Part model, mm, in its own coordinate system. A direction names the side the tool comes from. Coordinates: 2 decimals unless noted, no trailing zeros. Loops run counter-clockwise (first coordinate to the right, second up) from the corner with the lowest first, then second, coordinate; pieces in that order, holes last. Notation, with made-up numbers: (27, 35.25) - (62, 35.25) arc R22 cw to (62, 64.25) - close; hole circle Ø6 at (58.25, 54). An arc over 180 degrees is marked (long way). Use a Markdown table: item, result. Add a question column.
1. Wall check: probe 1 along X at (y, z) = (1.5, 0); probe 2 along Y at (x, z) = (5, 0.9); probe 3 along Y at (x, z) = (31.5, -2.6). Give the ranges that are in metal, low to high. Write a range as [from, to].
2. 3-axis set-ups, long thin cutter, end or side, ignore diameter. For faces 1 (the flat face through (16, 1, -3)), 2 (the flat face through (32, 3.5, 2)): which of +Z, -Z, +X, -X, +Y, -Y reach the whole face in a straight line?
3. Band-saw the part on C-C, the plane x = 12.5. Give the cut face in (y, z).
4. Band-saw the part on A-A, the plane z = 0. Give the cut face in (x, y).
5. Drop a flat-ended pin along its axis: pin 1 (1.8 mm diameter, centred on x = 32.5, z = 1, fed in from +Y). Give the stop position or say it passes through.
6. Band-saw the part on B-B, the plane y = 1. Give the cut face in (x, z), plus the area to 3 significant figures.
7. Pull direction Z, two halves, no side cores. Call faces 3 (the cylindrical face through (30.65, 1.77, 0.81)), 4 (the flat face through (-2, 4, 0)), 5 (the cylindrical face through (-2.93, 2.42, -0.65)), 6 (the cylindrical face through (-1.71, 2.03, -0.38)): pulls with the +Z half, pulls with the -Z half, needs draft (parallel to the pull), parting line crosses it, or undercut.
from build123d import *
from build123d.topology import SkipClean

# Parameters (mm, degrees)
EXTRUDE_1_DEPTH     = 3
SKETCH_2_R          = 3
EXTRUDE_2_DEPTH     = 0.5
SKETCH_3_R          = 3
EXTRUDE_3_DEPTH     = 1
SKETCH_4_R          = 1.75
CUT_EXTRUDE_1_DEPTH = 36.553340209


with BuildPart() as part:
    # Sketch 1 → Extrude 1 (new body)
    with BuildSketch(Plane(origin=(0, 0, 0), x_dir=(1, 0, 0), z_dir=(0, 1, 0))):
        with BuildLine():
            Line((0, 3), (32.2, 3))
            ThreePointArc((32.2, 3), (35.2, 0), (32.2, -3))
            Line((32.2, -3), (0, -3))
            ThreePointArc((0, -3), (-3, 0), (0, 3))
        make_face()
    extrude(amount=EXTRUDE_1_DEPTH)

    # Sketch 2 → Extrude 2 (add)
    with SkipClean():  # the faces are left unmerged after this step: merging them gives an invalid solid
        with BuildSketch(Plane(origin=(0, 3, 0), x_dir=(1, 0, 0), z_dir=(0, 1, 0))):
            with Locations(Location((32.2, 0, 0), (0, 0, 270))):
                Circle(SKETCH_2_R)
        extrude(amount=EXTRUDE_2_DEPTH)
    add(part.part.scale(1), mode=Mode.REPLACE)  # the faces are merged on a copy

    # Sketch 3 → Extrude 3 (add)
    with SkipClean():  # the faces are left unmerged after this step: merging them gives an invalid solid
        with BuildSketch(Plane(origin=(0, 3, 0), x_dir=(1, 0, 0), z_dir=(0, 1, 0))):
            with Locations(Location((0, 0, 0), (0, 0, 270))):
                Circle(SKETCH_3_R)
        extrude(amount=EXTRUDE_3_DEPTH)

    # Sketch 4 → Cut-Extrude 1 (cut, through all)
    with SkipClean():  # the faces are left unmerged after this step: merging them gives an invalid solid
        with BuildSketch(Plane(origin=(0, 4, 0), x_dir=(1, 0, 0), z_dir=(0, 1, 0))):
            with Locations(Location((0, 0, 0), (0, 0, 270))):
                Circle(SKETCH_4_R)
            with Locations(Location((32.2, 0, 0), (0, 0, 270))):
                Circle(SKETCH_4_R)
        extrude(amount=-CUT_EXTRUDE_1_DEPTH, mode=Mode.SUBTRACT)


solid = part.part
Geometry check:
| question | item | result |
|---|---|---|
| 1 | probe 1 | x = [-3, -1.75], [1.75, 30.45], [33.95, 35.2] |
| 1 | probe 2 | y = [0, 3] |
| 1 | probe 3 | y = [0, 3.5] |
| 2 | face 1 | -Z, +X, -X, +Y, -Y |
| 2 | face 2 | +Z, -Z, +X, +Y |
| 3 | outline | (0, -3) - (3, -3) - (3, 3) - (0, 3) - close |
| 4 | outline | (-3, 0) - (-1.75, 0) - (-1.75, 4) - (-3, 4) - close; (1.75, 0) - (30.45, 0) - (30.45, 3.5) - (29.2, 3.5) - (29.2, 3) - (3, 3) - (3, 4) - (1.75, 4) - close; (33.95, 0) - (35.2, 0) - (35.2, 3.5) - (33.95, 3.5) - close |
| 5 | pin 1 | stops at y = 3.5 |
| 6 | outline | (0, -3) - (32.2, -3) arc R3 ccw to (32.2, 3) - (0, 3) arc R3 ccw to start; hole circle Ø3.5 at (0, 0); hole circle Ø3.5 at (32.2, 0) |
| 6 | area | 202 mm^2 |
| 7 | face 3 | undercut |
| 7 | face 4 | needs draft |
| 7 | face 5 | parting line crosses it |
| 7 | face 6 | undercut |
